```python
from build123d import *

# Parameters (mm, degrees)
F0_W     = 25.4
F0_H     = 50.8
F0_W_2   = 20.32
F0_H_2   = 45.72
F1_DEPTH = 355.6
F2_R     = 2.5527
F3_DEPTH = 50.8
F4_R     = 2.5527
F5_DEPTH = 25.4


with BuildPart() as f1:
    # F0 (on Top) → F1 (new body)
    with BuildSketch(Plane.XY):
        with Locations((12.7, -25.4)):
            Rectangle(F0_W, F0_H)
        with Locations((12.7, -25.4)):
            Rectangle(F0_W_2, F0_H_2, mode=Mode.SUBTRACT)
    extrude(amount=F1_DEPTH)

    # F2 (on face) → F3 (cut)
    with BuildSketch(Plane.XZ.offset(50.8)):
        with Locations((12.7, 139.7)):
            Circle(F2_R)
        with Locations((12.7, 114.3)):
            Circle(F2_R)
        with Locations((12.7, 88.9)):
            Circle(F2_R)
        with Locations((12.7, 63.5)):
            Circle(F2_R)
        with Locations((12.7, 38.1)):
            Circle(F2_R)
        with Locations((12.7, 12.7)):
            Circle(F2_R)
        with Locations((12.7, 165.1)):
            Circle(F2_R)
        with Locations((12.7, 190.5)):
            Circle(F2_R)
        with Locations((12.7, 215.9)):
            Circle(F2_R)
        with Locations((12.7, 241.3)):
            Circle(F2_R)
    extrude(amount=-F3_DEPTH, mode=Mode.SUBTRACT)

    # F4 (on face) → F5 (cut)
    with BuildSketch(Plane.YZ.offset(25.4)):
        with Locations((-38.1, 38.1)):
            Circle(F4_R)
        with Locations((-12.7, 38.1)):
            Circle(F4_R)
        with Locations((-12.7, 12.7)):
            Circle(F4_R)
        with Locations((-38.1, 12.7)):
            Circle(F4_R)
        with Locations((-38.1, 92.075)):
            Circle(F4_R)
        with Locations((-12.7, 92.075)):
            Circle(F4_R)
    extrude(amount=-F5_DEPTH, mode=Mode.SUBTRACT)


solid = f1.part
```
CAD build for the part. Positions are in the model's coordinates, mm. A direction names the side the tool comes from. Coordinates: 2 decimals unless noted, no trailing zeros. Write each loop counter-clockwise with the first axis right and the second up, starting at its lowest first coordinate (ties: lowest second). Pieces come first, ordered by that corner, then holes. Notation, with made-up numbers: (-9, -39.75) -> (34, -39.75) arc R14 cw to (34, -31.75) -> close; hole circle Ø8 at (9.5, 32). An arc over 180 degrees is marked (long way). Use CSV: the item, a comma, the result in double quotes. Start each with the question number.
Item 1: Wall check: probe 1 along Y at (x, z) = (15, 153.5); probe 2 along X at (y, z) = (-19, 298.5); probe 3 along Z at (x, y) = (1.75, -38.1). Give the ranges that are in metal, low to high.
Item 2: Two-plate mould, pull along X, no slides. Class faces 3 (the flat face through (2.54, -26, 175)), 4 (the flat face through (2, -23, 0)), 5 (the flat face through (25.4, -26, 175)): +X half, -X half, draft (parallel to the pull), parting line (faces both ways), or undercut.
Item 3: Band-saw the part on B-B, the plane z = 295. Write the cut outline in (x, y).
Item 4: Band-saw the part on A-A, the plane y = -24. Write the cut outline in (x, z).
Item 5: Drop a flat-ended pin along its axis: P1, Ø6.5, axis at x = 12.7, z = 88.9, coming from the -Y side. Give the stop position or say it passes through.
Item 6: Tool access for faces 1 (the flat face through (13, -2.54, 175)), 2 (the flat face through (13, -50.8, 175)): list every direction of +Z, -Z, +X, -X, +Y, -Y with a clear straight run to the whole face (end or side of a thin tool).
Response values:
1,probe 1,"y = -50.8 to -48.26, -2.54 to 0"
1,probe 2,"x = 0 to 2.54, 22.86 to 25.4"
1,probe 3,"z = 0 to 10.15, 15.25 to 35.55, 40.65 to 89.52, 94.63 to 355.6"
2,face 3,"undercut"
2,face 4,"draft"
2,face 5,"+X half"
3,outline,"(0, -50.8) -> (25.4, -50.8) -> (25.4, 0) -> (0, 0) -> close; hole (2.54, -48.26) -> (22.86, -48.26) -> (22.86, -2.54) -> (2.54, -2.54) -> close"
4,outline,"(0, 0) -> (2.54, 0) -> (2.54, 355.6) -> (0, 355.6) -> close; (22.86, 0) -> (25.4, 0) -> (25.4, 355.6) -> (22.86, 355.6) -> close"
5,P1,"stops at y = -50.8"
6,face 1,"+Z, -Z"
6,face 2,"+Z, -Z, +X, -X, -Y"
